Source: CAD feature listing. Evaluate the final solid. Frame: model axes, mm. A direction names the side the tool comes from. Coordinates: 2 decimals unless noted, no trailing zeros. Write each loop counter-clockwise with the first axis right and the second up, starting at its lowest first coordinate (ties: lowest second). Pieces come first, ordered by that corner, then holes. Notation, with made-up numbers: M 30,28.25 L 84,28.25 A28 cw 84,50.25 Z; hole C -13,78.5 d10. An arc over 180 degrees is marked long. Write item = value, one per line. Start each with the question number.
1. Section query D-D (z = -85). Output: boundary loops of the cut face in (x, y).
2. Line query: line 1 along X through (y, z) = (11.5, 121); line 2 along Y through (x, z) = (80, 125); line 3 along Y through (x, z) = (-68.5, 15.5). Output: solid intervals per line, ascending.
3. Pin query (flat end, axial travel): pin 1 Ø12 at (x, y) = (62.5, 63) entering from +Z; pin 2 Ø18.5 at (y, z) = (43, -143.5) entering from -X; pin 3 Ø8 at (y, z) = (57.5, 8.5) entering from +X. Return the tip coordinate at first contact, or that it passes through.
4. Section query C-C (y = 39). Output: boundary loops of the cut face in (x, z) (3 decimals), then the cut area to 3 significant figures.
5. Pull-direction query (Z, two-part tool) for faces 1 (the face through (1.32, 50.26, -35.34)), 2 (the face through (-43.348, 50, -125)), 3 (the face through (80.28, 49.12, 105.02)); classes: pulls with the +Z half, pulls with the -Z half, needs draft (parallel to the pull), parting line crosses it, or undercut.
6. Access query for faces 4 (the face through (-60, 51, 99)), 5 (the face through (43.348, 50, -127)), 6 (the face through (1, 31.68, -53)). Directions: +Z, -Z, +X, -X, +Y, -Y. A direction counts if a zero-diameter tool reaches every point of the face in a straight line with its end or side. Return the directions, or none.
7. Section query A-A (x = -80). Output: boundary loops of the cut face in (y, z), then the cut area to 3 significant figures.
8. Section query B-B (z = 14). Output: boundary loops of the cut face in (x, y).
```python
from build123d import *

# Parameters (mm, degrees)
SKETCH2_W           = 200
SKETCH2_H           = 350
BOSS_EXTRUDE1_DEPTH = 100
CUT_EXTRUDE3_DEPTH  = 226
SKETCH5_W           = 97.727308895
SKETCH5_H           = 31.680459025
CUT_EXTRUDE4_DEPTH  = 284.94541729


with BuildPart() as part:
    # Sketch2 → Boss-Extrude1 (new body)
    with BuildSketch(Plane(origin=(0, 0, 0), x_dir=(1, 0, 0), z_dir=(0, 1, 0))):
        Rectangle(SKETCH2_W, SKETCH2_H)
    extrude(amount=BOSS_EXTRUDE1_DEPTH)

    # Sketch4 → Cut-Extrude3 (cut, through all)
    with BuildSketch(Plane(origin=(0, 100, 0), x_dir=(1, 0, 0), z_dir=(0, 1, 0))):
        with BuildLine():
            Line((100, 175), (43.347633031, 175))
            Line((43.347633031, 175), (43.347633031, 77.272691105))
            ThreePointArc((43.347633031, 77.272691105), (45.866803863, 67.555664213), (52.789694192, 60.286522394))
            ThreePointArc((52.789694192, 60.286522394), (87.404145859, 23.940813259), (100, -24.644321249))
            Line((100, -24.644321249), (100, 175))
        make_face()
        with BuildLine():
            Line((-43.347633031, 77.272691105), (-43.347633031, 175))
            Line((-43.347633031, 175), (-100, 175))
            Line((-100, 175), (-100, -24.644321206))
            ThreePointArc((-100, -24.644321206), (-87.404145849, 23.940813278), (-52.789694192, 60.286522394))
            ThreePointArc((-52.789694192, 60.286522394), (-45.866803863, 67.555664213), (-43.347633031, 77.272691105))
        make_face()
        with BuildLine():
            Line((60, -175), (60, -24.644321162))
            ThreePointArc((60, -24.644321162), (0, 35.355678838), (-60, -24.644321162))
            Line((-60, -24.644321162), (-60, -175))
            Line((-60, -175), (60, -175))
        make_face()
    extrude(amount=-CUT_EXTRUDE3_DEPTH, mode=Mode.SUBTRACT)

    # Sketch5 → Cut-Extrude4 (cut, through all)
    with BuildSketch(Plane(origin=(100, 0, 0), x_dir=(0, 0, -1), z_dir=(1, 0, 0))):
        with BuildLine():
            Line((-175, 100), (-175, 50))
            ThreePointArc((-175, 50), (-160.355339059, 85.355339059), (-125, 100))
            Line((-125, 100), (-175, 100))
        make_face()
        with BuildLine():
            ThreePointArc((-105, 50), (-125, 70), (-145, 50))
            Line((-145, 50), (-105, 50))
        make_face()
        with BuildLine():
            Line((-105, 50), (-145, 50))
            ThreePointArc((-145, 50), (-125, 30), (-105, 50))
        make_face()
        with BuildLine():
            ThreePointArc((-125, 0), (-160.355339059, 14.644660941), (-175, 50))
            Line((-175, 50), (-175, 0))
            Line((-175, 0), (-125, 0))
        make_face()
        with BuildLine():
            ThreePointArc((-83.15716493, 22.628899304), (-101.215078672, 6.019578022), (-125, 0))
            Line((-125, 0), (-24.644321162, 0))
            Line((-24.644321162, 0), (-24.644321162, 31.680459025))
            Line((-24.644321162, 31.680459025), (-66.420030902, 31.680459025))
            ThreePointArc((-66.420030902, 31.680459025), (-75.933999434, 29.272627817), (-83.15716493, 22.628899304))
        make_face()
        with BuildLine():
            Line((-124.644321162, 100), (-125, 100))
            ThreePointArc((-125, 100), (-101.215078672, 93.980421978), (-83.15716493, 77.371100696))
            ThreePointArc((-83.15716493, 77.371100696), (-75.933999434, 70.727372183), (-66.420030902, 68.319540975))
            Line((-66.420030902, 68.319540975), (-24.644321162, 68.319540975))
            Line((-24.644321162, 68.319540975), (-24.644321162, 100))
            Line((-24.644321162, 100), (-124.644321162, 100))
        make_face()
        Polygon((60.286522394, 100), (-24.644321162, 100), (-24.644321162, 68.319540975), (77.272691105, 68.319540975), (77.272691105, 100), align=None)
        Polygon((-24.644321162, 31.680459025), (-24.644321162, 0), (60.286522394, 0), (77.272691105, 0), (77.272691105, 31.680459025), align=None)
        with Locations((126.136345553, 15.840229513)):
            Rectangle(SKETCH5_W, SKETCH5_H)
        with Locations((126.136345553, 84.159770487)):
            Rectangle(SKETCH5_W, SKETCH5_H)
    extrude(amount=-CUT_EXTRUDE4_DEPTH, mode=Mode.SUBTRACT)


solid = part.part
```
Results are:
q1.outline = M -43.35,31.68 L 43.35,31.68 L 43.35,68.32 L -43.35,68.32 Z
q2.line_1 = -100 to -60, 60 to 100
q2.line_2 = 0 to 30, 70 to 100
q2.line_3 = 31.68 to 68.32
q3.pin_1 = 174.51
q3.pin_2 = -43.35
q3.pin_3 = 99.26
q4.outline = M -100,24.644 A100 ccw -52.79,-60.287 A20 cw -43.348,-77.273 L -43.348,-175 L 43.348,-175 L 43.348,-77.273 A20 cw 52.79,-60.287 A100 ccw 100,24.644 L 100,108.297 L 60,108.297 L 60,24.644 A60 cw -60,24.644 L -60,108.297 L -100,108.297 Z; M -100,141.703 L -60,141.703 L -60,173.775 L -100,173.775 Z; M 60,141.703 L 100,141.703 L 100,173.775 L 60,173.775 Z
q4.area = 28,300 mm^2
q5.face_1 = pulls with the +Z half
q5.face_2 = needs draft
q5.face_3 = undercut
q6.face_4 = +Z, +Y, -Y
q6.face_5 = -Z, +X, +Y, -Y
q6.face_6 = -Z, +X, -X, -Y
q7.outline = M 22.63,83.16 A20 cw 31.68,66.42 L 31.68,-35.36 L 68.32,-35.36 L 68.32,66.42 A20 cw 77.37,83.16 A50 ccw long Z; hole C 50,125 d40
q7.area = 10,700 mm^2
q8.outline = M -99.43,31.68 L -59.05,31.68 L -59.05,68.32 L -99.43,68.32 Z; M 59.05,31.68 L 99.43,31.68 L 99.43,68.32 L 59.05,68.32 Z
